from build123d import *

# Parameters (mm, degrees)
SKETCH_1_W             = 200
SKETCH_1_H             = 230.75
EXTRUDE_1_DEPTH        = 3
SKETCH_2_W             = 3
SKETCH_2_H             = 15
CUT_EXTRUDE_1_DEPTH    = 306.37610008
PATTERN_LINEAR_1_COUNT = 5
PATTERN_LINEAR_1_PITCH = 40
SKETCH_3_W             = 15
SKETCH_3_H             = 3
CUT_EXTRUDE_2_DEPTH    = 306.37610008
SKETCH_4_R             = 1
CUT_EXTRUDE_3_DEPTH    = 306.37610008
CUT_EXTRUDE_4_DEPTH    = 306.37610008
PATTERN_LINEAR_2_COUNT = 5
PATTERN_LINEAR_2_PITCH = 40
MIRROR_1_COPY_1_DEPTH  = 306.37610008
MIRROR_1_COPY_2_DEPTH  = 306.37610008
MIRROR_1_COPY_3_DEPTH  = 306.37610008
MIRROR_1_COPY_4_DEPTH  = 306.37610008
SKETCH_6_W             = 15
SKETCH_6_H             = 20
CUT_EXTRUDE_5_DEPTH    = 306.37610008


with BuildPart() as part:
    # 草图1 → 凸台-拉伸1 (new body)
    with BuildSketch(Plane(origin=(0, 0, 0), x_dir=(1, 0, 0), z_dir=(0, 1, 0))):
        with Locations((100, 115.375)):
            Rectangle(SKETCH_1_W, SKETCH_1_H)
    extrude(amount=EXTRUDE_1_DEPTH)

    # 草图2 → 切除-拉伸1 (cut, through all)
    with BuildSketch(Plane(origin=(0, 3, 0), x_dir=(1, 0, 0), z_dir=(0, 1, 0))):
        with Locations((1.5, 195)):
            Rectangle(SKETCH_2_W, SKETCH_2_H)
        with Locations((198.5, 195)):
            Rectangle(SKETCH_2_W, SKETCH_2_H)
    cut_extrude_1 = extrude(amount=-CUT_EXTRUDE_1_DEPTH, mode=Mode.SUBTRACT)

    # 阵列(线性)1: 切除-拉伸1 ×5
    with Locations(*[(0, 0, i * PATTERN_LINEAR_1_PITCH) for i in range(1, PATTERN_LINEAR_1_COUNT)]):
        add(cut_extrude_1, mode=Mode.SUBTRACT)

    # 草图3 → 切除-拉伸2 (cut, through all)
    with BuildSketch(Plane(origin=(0, 3, 0), x_dir=(1, 0, 0), z_dir=(0, 1, 0))):
        with Locations((27.5, 1.5)):
            Rectangle(SKETCH_3_W, SKETCH_3_H)
        with Locations((62.5, 1.5)):
            Rectangle(SKETCH_3_W, SKETCH_3_H)
        with Locations((137.5, 1.5)):
            Rectangle(SKETCH_3_W, SKETCH_3_H)
        with Locations((172.5, 1.5)):
            Rectangle(SKETCH_3_W, SKETCH_3_H)
    extrude(amount=-CUT_EXTRUDE_2_DEPTH, mode=Mode.SUBTRACT)

    # 草图4 → 切除-拉伸3 (cut, through all)
    with BuildSketch(Plane(origin=(0, 3, 0), x_dir=(1, 0, 0), z_dir=(0, 1, 0))):
        with Locations(Location((100, 2, 0), (0, 0, 270))):
            Circle(SKETCH_4_R)
        with Locations(Location((45, 2, 0), (0, 0, 270))):
            Circle(SKETCH_4_R)
        with Locations(Location((155, 2, 0), (0, 0, 270))):
            Circle(SKETCH_4_R)
    extrude(amount=-CUT_EXTRUDE_3_DEPTH, mode=Mode.SUBTRACT)

    # 草图5 → 切除-拉伸4 (cut, through all)
    with BuildSketch(Plane(origin=(0, 3, 0), x_dir=(1, 0, 0), z_dir=(0, 1, 0))):
        Polygon((5, 197.05), (7, 197.05), (7, 196), (10, 196), (10, 194), (7, 194), (7, 192.95), (5, 192.95), (5, 194), (3, 194), (3, 196), (5, 196), align=None)
    cut_extrude_4 = extrude(amount=-CUT_EXTRUDE_4_DEPTH, mode=Mode.SUBTRACT)

    # 阵列(线性)2: 切除-拉伸4 ×5
    with Locations(*[(0, 0, i * PATTERN_LINEAR_2_PITCH) for i in range(1, PATTERN_LINEAR_2_COUNT)]):
        add(cut_extrude_4, mode=Mode.SUBTRACT)

    # 镜向1: 切除-拉伸4 across plane
    add(cut_extrude_4.mirror(Plane.ZY.offset(-100)), mode=Mode.SUBTRACT)

    # 镜向1 copy 1 sketch → 镜向1 copy 1 (cut, through all)
    with BuildSketch(Plane(origin=(200, 3, 40), x_dir=(-1, 0, 0), z_dir=(0, 1, 0))):
        Polygon((5, -197.05), (7, -197.05), (7, -196), (10, -196), (10, -194), (7, -194), (7, -192.95), (5, -192.95), (5, -194), (3, -194), (3, -196), (5, -196), align=None)
    extrude(amount=-MIRROR_1_COPY_1_DEPTH, mode=Mode.SUBTRACT)

    # 镜向1 copy 2 sketch → 镜向1 copy 2 (cut, through all)
    with BuildSketch(Plane(origin=(200, 3, 80), x_dir=(-1, 0, 0), z_dir=(0, 1, 0))):
        Polygon((5, -197.05), (7, -197.05), (7, -196), (10, -196), (10, -194), (7, -194), (7, -192.95), (5, -192.95), (5, -194), (3, -194), (3, -196), (5, -196), align=None)
    extrude(amount=-MIRROR_1_COPY_2_DEPTH, mode=Mode.SUBTRACT)

    # 镜向1 copy 3 sketch → 镜向1 copy 3 (cut, through all)
    with BuildSketch(Plane(origin=(200, 3, 120), x_dir=(-1, 0, 0), z_dir=(0, 1, 0))):
        Polygon((5, -197.05), (7, -197.05), (7, -196), (10, -196), (10, -194), (7, -194), (7, -192.95), (5, -192.95), (5, -194), (3, -194), (3, -196), (5, -196), align=None)
    extrude(amount=-MIRROR_1_COPY_3_DEPTH, mode=Mode.SUBTRACT)

    # 镜向1 copy 4 sketch → 镜向1 copy 4 (cut, through all)
    with BuildSketch(Plane(origin=(200, 3, 160), x_dir=(-1, 0, 0), z_dir=(0, 1, 0))):
        Polygon((5, -197.05), (7, -197.05), (7, -196), (10, -196), (10, -194), (7, -194), (7, -192.95), (5, -192.95), (5, -194), (3, -194), (3, -196), (5, -196), align=None)
    extrude(amount=-MIRROR_1_COPY_4_DEPTH, mode=Mode.SUBTRACT)

    # 草图6 → 切除-拉伸5 (cut, through all)
    with BuildSketch(Plane(origin=(0, 3, 0), x_dir=(1, 0, 0), z_dir=(0, 1, 0))):
        with Locations((67.5, 72)):
            Rectangle(SKETCH_6_W, SKETCH_6_H)
        with Locations((132.5, 72)):
            Rectangle(SKETCH_6_W, SKETCH_6_H)
    extrude(amount=-CUT_EXTRUDE_5_DEPTH, mode=Mode.SUBTRACT)


solid = part.part
Input: part model. Units: mm. Frame: model coordinates. Coordinates: 2 decimals unless noted, no trailing zeros. Loops run counter-clockwise (first coordinate to the right, second up) from the corner with the lowest first, then second, coordinate; pieces in that order, holes last. Notation, with made-up numbers: (33, -22) -> (61, -22) arc R9 ccw to (61, -8) -> close; hole circle Ø7 at (51, 51.25). An arc over 180 degrees is marked (long way). Write each question's results on one line, items separated by ' | '. Start each with the question number.
Q1. Section A-A, the plane z = -199.5. Return the cut outline in (x, y), plus the area to 3 significant figures.
Q2. Ray query, line 1 (X direction, y = 2.95, z = -193.5); line 2 (Z direction, x = 59, y = 0.3); line 3 (Z direction, x = 155, y = 1.65). Return the intervals inside material, ascending. Write a range as from..to.
Q3. Section B-B, the plane y = 0.45. State how many separate pieces and enclosed holes the cut face has, plus the area to 3 significant figures.
Q4. Pin query (flat end, axial travel): pin 1 (1.2 mm diameter, centred on y = 1.5, z = -116.5, fed in from +X); pin 2 (0.6 mm diameter, centred on y = 1.5, z = -74.5, fed in from +X). Return the tip coordinate at first contact, or that it passes through.
Found:
1) outline: (3, 0) -> (197, 0) -> (197, 3) -> (3, 3) -> close | area: 582 mm2
2) line 1: 3..5, 7..193, 195..197 | line 2: -230.75..-3 | line 3: -230.75..-3, -1..0
3) separate pieces: 1 | enclosed holes: 5 | area: 44,700 mm2
4) pin 1: x = 197 | pin 2: x = 190
